Read the model definition and answer for the solid it produces. Units are mm, in the model's axes. A direction names the side the tool comes from. Give positions to 0.01 mm unless a question says otherwise; leave off trailing zeros. Write each loop counter-clockwise with the first axis right and the second up, starting at its lowest first coordinate (ties: lowest second). Pieces come first, ordered by that corner, then holes. Notation, with made-up numbers: (18, 18.25) -> (75, 18.25) arc R12 cw to (75, 23.25) -> close; hole circle Ø6 at (65.25, 64.25). An arc over 180 degrees is marked (long way). Put each result on its own line as item: value. Start each with the question number.
from build123d import *

# Parameters (mm, degrees)
F0_W     = 32
F0_H     = 38
F0_R     = 1.1
F0_R_2   = 4.5
F1_DEPTH = 25
F2_W     = 20
F2_H     = 22
F3_DEPTH = 38.001
F5_DEPTH = 18


with BuildPart() as f1:
    # F0 (on Top) → F1 (new body)
    with BuildSketch(Plane.XY):
        with Locations((0, -11)):
            Rectangle(F0_W, F0_H)
        with Locations((-13.5, -28)):
            Circle(F0_R, mode=Mode.SUBTRACT)
        with Locations((13.5, -28)):
            Circle(F0_R, mode=Mode.SUBTRACT)
        with Locations((-13.5, -1)):
            Circle(F0_R, mode=Mode.SUBTRACT)
        Circle(F0_R_2, mode=Mode.SUBTRACT)
        with Locations((13.5, -1)):
            Circle(F0_R, mode=Mode.SUBTRACT)
    extrude(amount=F1_DEPTH)

    # F2 (on face) → F3 (cut, through all)
    with BuildSketch(Plane(origin=(0, 8, 0), x_dir=(-1, 0, 0), z_dir=(0, 1, 0))):
        with Locations((0, 14)):
            Rectangle(F2_W, F2_H)
    extrude(amount=-F3_DEPTH, mode=Mode.SUBTRACT)

    # F4 (on face) → F5 (cut)
    with BuildSketch(Plane(origin=(0, 0, 0), x_dir=(1, 0, 0), z_dir=(0, 0, -1))):
        with BuildLine():
            Line((16, -1.44077), (16, 3.44077))
            ThreePointArc((16, 3.44077), (10.006097, 1), (16, -1.44077))
        make_face()
        with BuildLine():
            ThreePointArc((-16, -2.520859), (-9.181847, 1), (-16, 4.520859))
            Line((-16, 4.520859), (-16, -2.520859))
        make_face()
        with BuildLine():
            ThreePointArc((10.304378, 30), (11.064189, 25.122705), (16, 25.178298))
            Line((16, 25.178298), (16, 30))
            Line((16, 30), (10.304378, 30))
        make_face()
        with BuildLine():
            Line((-16, 30), (-16, 24.341244))
            ThreePointArc((-16, 24.341244), (-10.578677, 24.667979), (-9.545699, 30))
            Line((-9.545699, 30), (-16, 30))
        make_face()
    extrude(amount=-F5_DEPTH, mode=Mode.SUBTRACT)


solid = f1.part
1) A cutting plane is placed at C-C on y = -26. Give the vertices of the cut face in (x, z), and give its area (3 significant figures).
2) For faces 4 (the face through (10.539, -2.854, 8.874)), 5 (the face through (0, -11, 3)), 6 (the face through (12.4, -1, 21.5)), determine the directions among +Z, -Z, +X, -X, +Y, -Y from which every point of the face is accessible in a straight line to the end or side of a thin tool.
3) A cutting plane is placed at A-A on z = 21.5. Give the vertices of the cut face in (x, y), and give its area (3 significant figures).
4) For a pull along Y with two mould halves and no side action, classify faces 1 (the face through (-13, -26.8, 18)), 2 (the face through (12.014, -24.535, 8.874)), 3 (the face through (-13, -30, 21)) as pulls with the +Y half, pulls with the -Y half, needs draft (parallel to the pull), parting line crosses it, or undercut.
5) Each of these flat-tipped pins is pushed along its axis until it touches: pin 1 Ø1.5 at (x, z) = (-7.5, 5.5) entering from +Y; pin 2 Ø6.5 at (x, y) = (13.5, -1) entering from +Z; pin 3 Ø2.5 at (x, y) = (-13.5, -1) entering from -Z; pin 4 Ø6 at (x, y) = (0.5, -5.5) entering from +Z. Where does it stop, or does it pass through?
6) A cutting plane is placed at D-D on x = 13.5. Give the vertices of the cut face in (y, z), and give its area (3 significant figures).
7) Straight lines are drawn through the part: line 1 (X direction, y = -28, z = 21.25); line 2 (Y direction, x = 0, z = 1.85); line 3 (X direction, y = 4, z = 13.5). For each, find the intervals that lie inside material, in ascending order. Write a range as [from, to].
8) A cutting plane is placed at B-B on x = 0. Give the vertices of the cut face in (y, z).
Results found:
1. outline: (-16, 18) -> (-10, 18) -> (-10, 25) -> (-16, 25) -> close; (-9.55, 0) -> (10.3, 0) -> (10.3, 18) -> (16, 18) -> (16, 25) -> (10, 25) -> (10, 3) -> (-9.55, 3) -> close
1. area: 148 mm²
2. face 4: -Z
2. face 5: +Z, +Y, -Y
2. face 6: +Z, -Z
3. outline: (-16, -30) -> (-10, -30) -> (-10, 8) -> (-16, 8) -> close; (10, -30) -> (16, -30) -> (16, 8) -> (10, 8) -> close; hole circle Ø2.2 at (-13.5, -28); hole circle Ø2.2 at (-13.5, -1); hole circle Ø2.2 at (13.5, -28); hole circle Ø2.2 at (13.5, -1)
3. area: 441 mm²
4. face 1: needs draft
4. face 2: undercut
4. face 3: pulls with the -Y half
5. pin 1: passes through
5. pin 2: stops at z = 25
5. pin 3: stops at z = 18
5. pin 4: stops at z = 3
6. outline: (-30, 18) -> (-29.1, 18) -> (-29.1, 25) -> (-30, 25) -> close; (-26.9, 18) -> (-24.23, 18) -> (-24.23, 0) -> (-4.49, 0) -> (-4.49, 18) -> (-2.1, 18) -> (-2.1, 25) -> (-26.9, 25) -> close; (0.1, 18) -> (2.49, 18) -> (2.49, 0) -> (8, 0) -> (8, 25) -> (0.1, 25) -> close
6. area: 690 mm²
7. line 1: x = [-16, -14.6], [-12.4, -10], [10, 12.4], [14.6, 16]
7. line 2: y = [-30, -4.5], [4.5, 8]
7. line 3: x = [-16, -10], [10, 16]
8. outline: (-30, 0) -> (-4.5, 0) -> (-4.5, 3) -> (-30, 3) -> close; (4.5, 0) -> (8, 0) -> (8, 3) -> (4.5, 3) -> close
